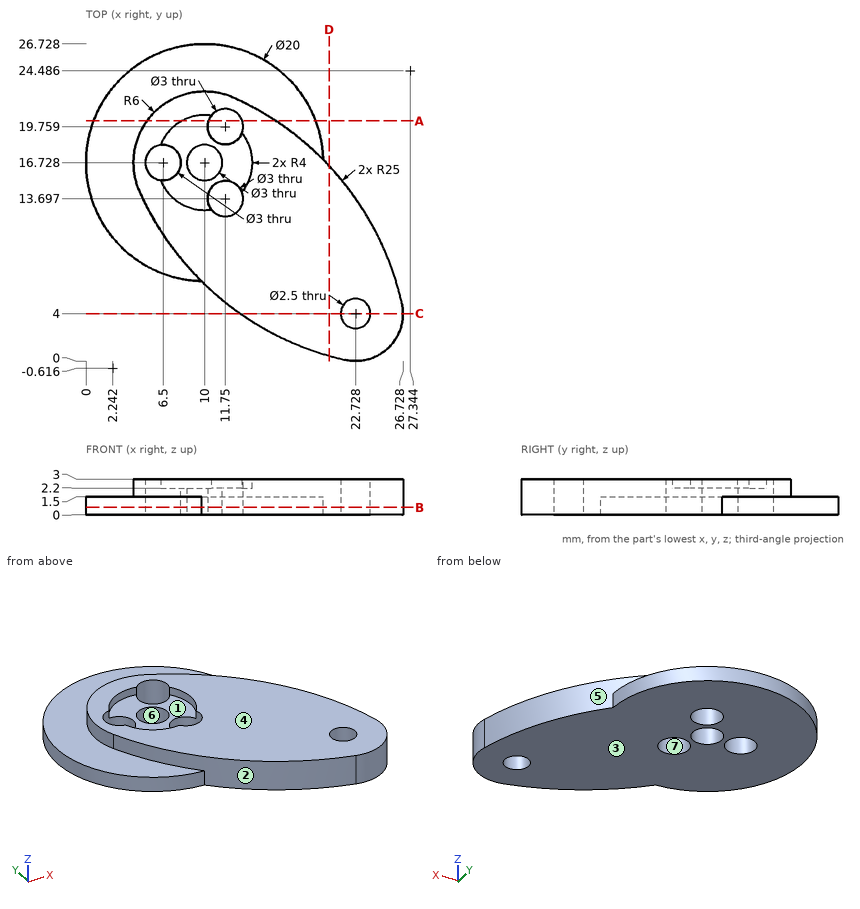
Drawing for the job (mm, zero at the part's lowest x, y, z). A direction names the side the tool comes from. Round coordinates to 2 decimals unless told otherwise and drop trailing zeros. Write each loop counter-clockwise with the first axis right and the second up, starting at its lowest first coordinate (ties: lowest second). Pieces come first, ordered by that corner, then holes. Notation, with made-up numbers: M 76.5,83.5 L 107.5,83.5 A11 cw 107.5,92.5 Z; hole C 70.5,-18 d11. An arc over 180 degrees is marked long. Answer as a JSON object with one key per item and string values. Group by question number.
(1) Which spindle directions (+Z, -Z, +X, -X, +Y, -Y) get a long thin tool onto all of the face, cutting with end or side? Do the marked faces 1, 2 and 3. Say none if no direction does.
(2) Cut at B-B (z = 0.6). Give the number of separate pieces and of enclosed holes in the cut face.
(3) Cut at A-A (y = 20.25). Give the cut face in (x, z).
(4) Cut at C-C (y = 4). Give the cut face in (x, z) (1 decimal).
(5) Mould opens along Y. For the marked faces 4, 5, 6 and 7 say: pulls with the +Y half, pulls with the -Y half, needs draft (parallel to the pull), parting line crosses it, or undercut.
(6) Cut at D-D (x = 20.5). Give the cut face in (y, z).
(7) Drill centre lines: L1, parallel to X at y = 18, z = 1.85 (1 decimal); L2, parallel to Y at x = 11.75, z = 2.1 (1 decimal); L3, parallel to Y at x = 11.75, z = 0.6 (1 decimal). Where is each one in solid material? Low to high.
(8) Flat gauge pins, fed straight in: pin 1 (4 mm diameter, centred on x = 9, y = 18, fed in from +Z); pin 2 (1.5 mm diameter, centred on x = 11.5, z = 1.5, fed in from +Y); pin 3 (1.5 mm diameter, centred on y = 22, z = 2, fed in from +X). Where does each tip first touch, or does it go through?
Responses:
{
 "1": {"face 1": "+Z", "face 2": "+Z, -X, -Y", "face 3": "-Z, +X, -X, +Y, -Y"},
 "2": {"separate pieces": "1", "enclosed holes": "5"},
 "3": {"outline": "M 0.64,0 L 10.33,0 L 10.33,2.2 L 8.1,2.2 L 8.1,3 L 5.14,3 L 5.14,1.5 L 0.64,1.5 Z; M 13.17,0 L 19.36,0 L 19.36,1.5 L 16.01,1.5 L 16.01,3 L 13.17,3 Z"},
 "4": {"outline": "M 13,0 L 21.5,0 L 21.5,3 L 13,3 Z; M 24,0 L 26.7,0 L 26.7,3 L 24,3 Z"},
 "5": {"face 4": "needs draft", "face 5": "pulls with the +Y half", "face 6": "undercut", "face 7": "undercut"},
 "6": {"outline": "M 0.44,0 L 16.46,0 L 16.46,3 L 0.44,3 Z"},
 "7": {"L1": "x = 4.1 to 5.7, 7.3 to 9.2, 10.8 to 18.9", "L2": "y = 4.9 to 12.2, 15.2 to 18.3, 21.3 to 22.5", "L3": "y = 4.9 to 12.2, 15.2 to 18.3, 21.3 to 26.6"},
 "8": {"pin 1": "stops at z = 2.2", "pin 2": "stops at y = 26.7", "pin 3": "stops at x = 18.82"}
}
